Source: CAD feature listing. Evaluate the final solid. Frame: model axes, mm. Face numbers are marked on the shaded views. A direction names the side the tool comes from. Give positions to 0.01 mm unless a question says otherwise; leave off trailing zeros. Write each loop counter-clockwise with the first axis right and the second up, starting at its lowest first coordinate (ties: lowest second). Pieces come first, ordered by that corner, then holes. Notation, with made-up numbers: (-13, 76) -> (28, 76) arc R36 ccw to (28, 110) -> close; hole circle Ø4 at (23.25, 31.25). An arc over 180 degrees is marked (long way). Answer as a JSON object with one key per item and string values. Group by question number.
Item 1: First-contact query: pin 1 Ø11 at (x, z) = (-16, -83.5) entering from -Y; pin 2 Ø2.5 at (x, z) = (-3, -83) entering from -Y; pin 3 Ø2 at (x, y) = (-6, 1) entering from +Z; pin 4 Ø5 at (x, y) = (-20, 5.5) entering from +Z. Flat tips, straight axial feed; report the tip coordinate or a pass-through.
Item 2: Section query A-A on x = -4. Return the cut outline in (y, z).
Item 3: Access query for the marked faces 4 and 5. Directions: +Z, -Z, +X, -X, +Y, -Y. A direction counts if a zero-diameter tool reaches every point of the face in a straight line with its end or side. Return the directions, or none.
Item 4: Section query D-D on x = -25. Return the cut outline in (y, z), plus the area to 3 significant figures.
Item 5: Pull-direction query (Z, two-part tool) for the marked faces 1, 2 and 3; classes: pulls with the +Z half, pulls with the -Z half, needs draft (parallel to the pull), parting line crosses it, or undercut.
Item 6: Section query C-C on y = 9. Give the number of separate pieces and of enclosed holes in the cut face, plus the area to 3 significant figures.
Item 7: Ray query, probe 1 along Z at (x, y) = (-4, 1.75); probe 2 along Z at (x, y) = (-15, 4.5); probe 3 along Z at (x, y) = (-13, 3). Return the intervals inside material, ascending. Write a range as from..to.
from build123d import *

# Parameters (mm, degrees)
BOSS_EXTRUDE1_DEPTH                                 = 10
CHAMFER1_SIZE                                       = 5
CHAMFER2_SIZE                                       = 2.5
FILLET1_R                                           = 2.5
CBORE_FOR_M5_HEX_SOCKET_HEAD_CAP_SCREW5_D           = 5.5
CBORE_FOR_M5_HEX_SOCKET_HEAD_CAP_SCREW5_DEPTH       = 10
CBORE_FOR_M5_HEX_SOCKET_HEAD_CAP_SCREW5_CBORE_D     = 10
CBORE_FOR_M5_HEX_SOCKET_HEAD_CAP_SCREW5_CBORE_DEPTH = 5.4
CBORE_FOR_M5_HEX_SOCKET_HEAD_CAP_SCREW5_TIP         = 1.652366702


# Some blends are built 0.0001 mm under size
with BuildPart() as part:
    # Sketch2 → Boss-Extrude1 (new body)
    with BuildSketch(Plane(origin=(0, 0, 0), x_dir=(1, 0, 0), z_dir=(0, 1, 0))):
        Polygon((0, 59.135462652), (-14.95, 59.135462652), (-14.95, 29.135462652), (-10.95, 29.135462652), (-10.95, 14.135462652), (-8.45, 14.135462652), (-8.45, 0), (-18.45, 0), (-35, 64.135462652), (-35, 89.135462652), (0, 89.135462652), align=None)
    extrude(amount=BOSS_EXTRUDE1_DEPTH)

    # Chamfer1
    chamfer1_edges = [part.edges().sort_by_distance(p)[0] for p in [
        (-14.95, 5, -59.135462652),
    ]]
    chamfer(chamfer1_edges, length=CHAMFER1_SIZE)

    # Chamfer2
    chamfer2_edges = [part.edges().sort_by_distance(p)[0] for p in [
        (-10.95, 5, -14.135462652),
        (-14.95, 5, -29.135462652),
    ]]
    chamfer(chamfer2_edges, length=CHAMFER2_SIZE - 0.0001)  # a hair under: the kernel refuses the full size

    # Fillet1
    # the kernel refuses this fillet: 2.5 mm, written as the material it takes off along each edge
    with BuildSketch(Plane(origin=(0, -6.25, -89.135462652), x_dir=(0, 0, 1), z_dir=(0, 1, 0)), Plane(origin=(-35, -6.25, -89.135462652), x_dir=(1, 0, 0), z_dir=(0, 1, 0)), Plane(origin=(0, -6.25, -59.135462652), x_dir=(-1, 0, 0), z_dir=(0, 1, 0))) as fillet1_piece_1:
        with BuildLine():
            CenterArc((FILLET1_R, -FILLET1_R), FILLET1_R, 90, 90)
            Line((0, -FILLET1_R), (-FILLET1_R * 0.02, -FILLET1_R))
            Line((-FILLET1_R * 0.02, -FILLET1_R), (-FILLET1_R * 0.02, FILLET1_R * 0.02))
            Line((-FILLET1_R * 0.02, FILLET1_R * 0.02), (FILLET1_R, FILLET1_R * 0.02))
            Line((FILLET1_R, FILLET1_R * 0.02), (FILLET1_R, 0))
        make_face()
    extrude(amount=22.5, mode=Mode.SUBTRACT)
    with BuildSketch(Plane(origin=(-8.45, -6.25, 0), x_dir=(0, 0, -1), z_dir=(0, 1, 0))) as fillet1_piece_2:
        with BuildLine():
            CenterArc((FILLET1_R, FILLET1_R), FILLET1_R, 180, 90)
            Line((0, FILLET1_R), (-FILLET1_R * 0.02, FILLET1_R))
            Line((-FILLET1_R * 0.02, FILLET1_R), (-FILLET1_R * 0.02, -FILLET1_R * 0.02))
            Line((-FILLET1_R * 0.02, -FILLET1_R * 0.02), (FILLET1_R, -FILLET1_R * 0.02))
            Line((FILLET1_R, -FILLET1_R * 0.02), (FILLET1_R, 0))
        make_face()
    extrude(amount=22.5, mode=Mode.SUBTRACT)
    with BuildSketch(Plane(origin=(-18.45, -4.84193858, 0), x_dir=(-0.24986263082994187, 0, -0.9682812947252158), z_dir=(0, 1, 0))) as fillet1_piece_3:
        with BuildLine():
            CenterArc((FILLET1_R * 0.774710172815, -FILLET1_R), FILLET1_R, 90, 75.530616462)
            Line((-FILLET1_R * 0.19357112191, -FILLET1_R * 0.75013736917), (-FILLET1_R * 0.212936747805, -FILLET1_R * 0.745140116553))
            Line((-FILLET1_R * 0.212936747805, -FILLET1_R * 0.745140116553), (-FILLET1_R * 0.0154942034563, FILLET1_R * 0.02))
            Line((-FILLET1_R * 0.0154942034563, FILLET1_R * 0.02), (FILLET1_R * 0.774710172815, FILLET1_R * 0.02))
            Line((FILLET1_R * 0.774710172815, FILLET1_R * 0.02), (FILLET1_R * 0.774710172815, 0))
        make_face()
    extrude(amount=19.68387716, mode=Mode.SUBTRACT)
    with BuildSketch(Plane(origin=(-10.95, -5.728328721, -29.135462652), x_dir=(-1, 0, 0), z_dir=(0, 1, 0))) as fillet1_piece_4:
        with BuildLine():
            CenterArc((2.5, 2.291331488), FILLET1_R, 180, 66.424322091)
            Line((0, 2.291331488), (-0.05, 2.291331488))
            Line((-0.05, 2.291331488), (-0.05, 0))
            Line((-0.05, 0), (0, -0.05))
            ThreePointArc((0, -0.05), (0.75005, -0.05), (1.480102, -0.04582663))
            Line((1.480102, -0.04582663), (1.5001, 0))
        make_face()
    extrude(amount=21.456657442, mode=Mode.SUBTRACT)

    # CBORE for M5 Hex Socket Head Cap Screw5
    with Locations(Plane(origin=(0, 0, 0), x_dir=(-1, 0, 0), z_dir=(0, -1, 0))):
        with Locations((4, 81.635462652), (15, 81.635462652)):
            CounterBoreHole(CBORE_FOR_M5_HEX_SOCKET_HEAD_CAP_SCREW5_D / 2, CBORE_FOR_M5_HEX_SOCKET_HEAD_CAP_SCREW5_CBORE_D / 2, CBORE_FOR_M5_HEX_SOCKET_HEAD_CAP_SCREW5_CBORE_DEPTH, depth=CBORE_FOR_M5_HEX_SOCKET_HEAD_CAP_SCREW5_DEPTH)
            with Locations((0, 0, -(CBORE_FOR_M5_HEX_SOCKET_HEAD_CAP_SCREW5_DEPTH + CBORE_FOR_M5_HEX_SOCKET_HEAD_CAP_SCREW5_TIP / 2))):  # 118° drill point
                Cone(0, CBORE_FOR_M5_HEX_SOCKET_HEAD_CAP_SCREW5_D / 2, CBORE_FOR_M5_HEX_SOCKET_HEAD_CAP_SCREW5_TIP, mode=Mode.SUBTRACT)


solid = part.part
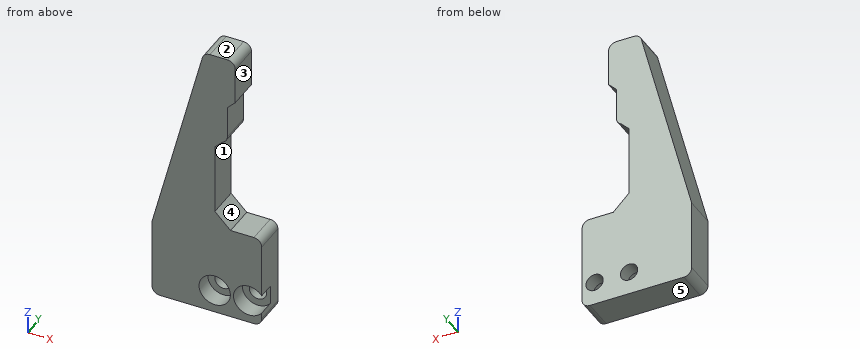
Worked answers:
{
 "1": {"pin 1": "y = 0", "pin 2": "y = 5.4", "pin 3": "z = -59.14", "pin 4": "z = -0.2"},
 "2": {"outline": "(0, -89.14) -> (10, -89.14) -> (10, -84.39) -> (5.4, -84.39) -> (5.4, -86.64) -> (0, -86.64) -> close; (0, -76.64) -> (5.4, -76.64) -> (5.4, -78.89) -> (10, -78.89) -> (10, -59.14) -> (0, -59.14) -> close"},
 "3": {"face 4": "+X, +Y, -Y", "face 5": "-Z, +X, -X, +Y, -Y"},
 "4": {"outline": "(0, -89.14) -> (10, -89.14) -> (10, -25.38) -> (0, -25.38) -> close", "area": "638 mm^2"},
 "5": {"face 1": "undercut", "face 2": "pulls with the +Z half", "face 3": "needs draft"},
 "6": {"separate pieces": "1", "enclosed holes": "2", "area": "1,820 mm^2"},
 "7": {"probe 1": "-89.14..-86.64, -76.64..-59.14", "probe 2": "-89.14..-86.64, -76.64..0", "probe 3": "-89.14..-86.22, -77.05..-56.09, -29.69..0"}
}
